For this review, take the finished solid that the model builds, in its own axes (mm). Face numbers are marked on the shaded views. Coordinates: 2 decimals unless noted, no trailing zeros. Loops run counter-clockwise (first coordinate to the right, second up) from the corner with the lowest first, then second, coordinate; pieces in that order, holes last.
1. Take a section at B-B, the plane z = -2.5. State the section outline as (x, y) points, then the cut area to 3 significant figures.
2. Mouldability with a two-part tool opening along Z and no side actions: class the marked faces 1 and 2 as pulls with the +Z half, pulls with the -Z half, needs draft (parallel to the pull), parting line crosses it, or undercut.
3. To check wall thickness, follow probe 1 along X at (y, z) = (0.15, -2); probe 2 along Z at (x, y) = (-3.5, 0.1); probe 3 along Y at (x, z) = (1.75, -2). State the ranges of each line that lie inside material, in increasing order.
4. Clearance check with a flat-ended pin moving along its axis: P1, Ø1, axis at x = -1.5, z = 6, coming from the +Y side. State where the tip first meets the part, or that it passes through.
5. Take a section at A-A, the plane x = -1. State the section outline as (y, z) points, then the cut area to 4 significant figures.
```python
from build123d import *

# Parameters (mm, degrees)
F1_DEPTH = 0.75
F2_DEPTH = 0.75
F3_DEPTH = 0.25


with BuildPart() as f1:
    # F0 (on Front) → F1 (new body)
    with BuildSketch(Plane.XZ):
        with BuildLine():
            Line((3.85, 7.75), (-3.85, 7.75))
            ThreePointArc((-3.85, 7.75), (-3.9207106781, 7.7207106781), (-3.95, 7.65))
            Line((-3.95, 7.65), (-3.95, -7.65))
            ThreePointArc((-3.95, -7.65), (-3.9207106781, -7.7207106781), (-3.85, -7.75))
            Line((-3.85, -7.75), (3.85, -7.75))
            ThreePointArc((3.85, -7.75), (3.9207106781, -7.7207106781), (3.95, -7.65))
            Line((3.95, -7.65), (3.95, 7.65))
            ThreePointArc((3.95, 7.65), (3.9207106781, 7.7207106781), (3.85, 7.75))
        make_face()
        with BuildLine():
            ThreePointArc((-3.7, 7.4), (-3.6707106781, 7.4707106781), (-3.6, 7.5))
            Line((-3.6, 7.5), (3.6, 7.5))
            ThreePointArc((3.6, 7.5), (3.6707106781, 7.4707106781), (3.7, 7.4))
            Line((3.7, 7.4), (3.7, -7.4))
            ThreePointArc((3.7, -7.4), (3.6707106781, -7.4707106781), (3.6, -7.5))
            Line((3.6, -7.5), (-3.6, -7.5))
            ThreePointArc((-3.6, -7.5), (-3.6707106781, -7.4707106781), (-3.7, -7.4))
            Line((-3.7, -7.4), (-3.7, 7.4))
        make_face(mode=Mode.SUBTRACT)
        with BuildLine():
            Line((3.6, 7.5), (-3.6, 7.5))
            ThreePointArc((-3.6, 7.5), (-3.6707106781, 7.4707106781), (-3.7, 7.4))
            Line((-3.7, 7.4), (-3.7, -7.4))
            ThreePointArc((-3.7, -7.4), (-3.6707106781, -7.4707106781), (-3.6, -7.5))
            Line((-3.6, -7.5), (3.6, -7.5))
            ThreePointArc((3.6, -7.5), (3.6707106781, -7.4707106781), (3.7, -7.4))
            Line((3.7, -7.4), (3.7, 7.4))
            ThreePointArc((3.7, 7.4), (3.6707106781, 7.4707106781), (3.6, 7.5))
        make_face()
    extrude(amount=F1_DEPTH)

    # F0 (on Front) → F2 (join)
    with BuildSketch(Plane.XZ):
        with BuildLine():
            Line((3.85, 7.75), (-3.85, 7.75))
            ThreePointArc((-3.85, 7.75), (-3.9207106781, 7.7207106781), (-3.95, 7.65))
            Line((-3.95, 7.65), (-3.95, -7.65))
            ThreePointArc((-3.95, -7.65), (-3.9207106781, -7.7207106781), (-3.85, -7.75))
            Line((-3.85, -7.75), (3.85, -7.75))
            ThreePointArc((3.85, -7.75), (3.9207106781, -7.7207106781), (3.95, -7.65))
            Line((3.95, -7.65), (3.95, 7.65))
            ThreePointArc((3.95, 7.65), (3.9207106781, 7.7207106781), (3.85, 7.75))
        make_face()
        with BuildLine():
            ThreePointArc((-3.7, 7.4), (-3.6707106781, 7.4707106781), (-3.6, 7.5))
            Line((-3.6, 7.5), (3.6, 7.5))
            ThreePointArc((3.6, 7.5), (3.6707106781, 7.4707106781), (3.7, 7.4))
            Line((3.7, 7.4), (3.7, -7.4))
            ThreePointArc((3.7, -7.4), (3.6707106781, -7.4707106781), (3.6, -7.5))
            Line((3.6, -7.5), (-3.6, -7.5))
            ThreePointArc((-3.6, -7.5), (-3.6707106781, -7.4707106781), (-3.7, -7.4))
            Line((-3.7, -7.4), (-3.7, 7.4))
        make_face(mode=Mode.SUBTRACT)
    extrude(amount=F2_DEPTH)

    # F0 (on Front) → F3 (join)
    with BuildSketch(Plane.XZ):
        with BuildLine():
            Line((3.85, 7.75), (-3.85, 7.75))
            ThreePointArc((-3.85, 7.75), (-3.9207106781, 7.7207106781), (-3.95, 7.65))
            Line((-3.95, 7.65), (-3.95, -7.65))
            ThreePointArc((-3.95, -7.65), (-3.9207106781, -7.7207106781), (-3.85, -7.75))
            Line((-3.85, -7.75), (3.85, -7.75))
            ThreePointArc((3.85, -7.75), (3.9207106781, -7.7207106781), (3.95, -7.65))
            Line((3.95, -7.65), (3.95, 7.65))
            ThreePointArc((3.95, 7.65), (3.9207106781, 7.7207106781), (3.85, 7.75))
        make_face()
        with BuildLine():
            ThreePointArc((-3.7, 7.4), (-3.6707106781, 7.4707106781), (-3.6, 7.5))
            Line((-3.6, 7.5), (3.6, 7.5))
            ThreePointArc((3.6, 7.5), (3.6707106781, 7.4707106781), (3.7, 7.4))
            Line((3.7, 7.4), (3.7, -7.4))
            ThreePointArc((3.7, -7.4), (3.6707106781, -7.4707106781), (3.6, -7.5))
            Line((3.6, -7.5), (-3.6, -7.5))
            ThreePointArc((-3.6, -7.5), (-3.6707106781, -7.4707106781), (-3.7, -7.4))
            Line((-3.7, -7.4), (-3.7, 7.4))
        make_face(mode=Mode.SUBTRACT)
    extrude(amount=-F3_DEPTH)


solid = f1.part
```
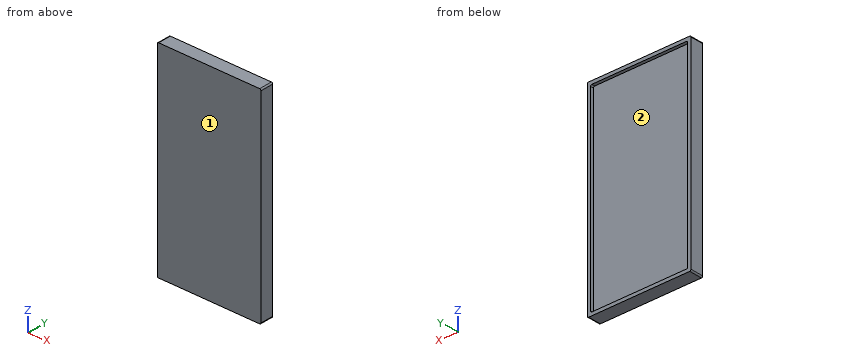
Results list:
1. outline: (-3.95, -0.75) - (3.95, -0.75) - (3.95, 0.25) - (3.7, 0.25) - (3.7, 0) - (-3.7, 0) - (-3.7, 0.25) - (-3.95, 0.25) - close
1. area: 6.05 mm2
2. face 1: needs draft
2. face 2: undercut
3. probe 1: x = -3.95 to -3.7, 3.7 to 3.95
3. probe 2: z = -7.75 to -7.5, 7.5 to 7.75
3. probe 3: y = -0.75 to 0
4. P1: stops at y = 0
5. outline: (-0.75, -7.75) - (0.25, -7.75) - (0.25, -7.5) - (0, -7.5) - (0, 7.5) - (0.25, 7.5) - (0.25, 7.75) - (-0.75, 7.75) - close
5. area: 11.75 mm2
